Could you check a few things on this model? Use its own coordinates, in mm. Face numbers are marked on the shaded views. A direction names the side the tool comes from. Give positions to 0.01 mm unless a question says otherwise; leave off trailing zeros. Loops run counter-clockwise (first coordinate to the right, second up) from the corner with the lowest first, then second, coordinate; pieces in that order, holes last. Notation, with made-up numbers: (63, -5.75) -> (96, -5.75) arc R17 ccw to (96, -0.75) -> close; hole circle Ø1 at (35, 51.25). An arc over 180 degrees is marked (long way). Write item = value, one per line. Start each with the question number.
1) I'm going to push flat-ended pins straight in: pin 1 Ø3 at (x, z) = (2, -6) entering from +Y; pin 2 Ø2 at (y, z) = (2.5, 2) entering from +X; pin 3 Ø4 at (x, z) = (0.5, 3) entering from +Y. Where does each tip first touch, or does it pass through?
2) I want a section at B-B (x = 0). List the corners of the cut face in (y, z) for me (3 decimals).
3) I want a section at A-A (z = 1). List the corners of the cut face in (x, y) for me (3 decimals), and give its area (3 significant figures).
4) I need wall thicknesses on probe 1 along Y at (x, z) = (0, -0.5) (3 decimals); probe 2 along Z at (x, y) = (-2.5, -2.25); probe 3 along X at (y, z) = (0, 3.5). Which ranges of each line are inside material? Lowest first, please. Write a range as from..to.
5) On a 3-axis mill with a long thin cutter (end or side, diameter ignored), from which of +Z, -Z, +X, -X, +Y, -Y can I reach the whole of each face in a straight line? I mean the marked faces 1, 2 and 3. Say none if no direction works.
6) I want a section at D-D (z = -6). List the corners of the cut face in (x, y) for me (3 decimals), and give its area (3 significant figures).
7) If we mould it in two halves opening along Y, with no side actions, what happens to the marked faces 4, 5 and 6? For each: +Y half, -Y half, draft (parallel to the pull), parting line (faces both ways), or undercut.
8) I want a section at C-C (x = 2.75). List the corners of the cut face in (y, z) for me.
from build123d import *

# Parameters (mm, degrees)
SALIENTE_EXTRUIR1_DEPTH = 3
CROQUIS5_R              = 2.9
SALIENTE_EXTRUIR2_DEPTH = 7.5
CROQUIS4_R              = 0.875
CORTAR_EXTRUIR1_DEPTH   = 10.5


with BuildPart() as part:
    # Croquis1 → Saliente-Extruir1 (new body)
    with BuildSketch(Plane.XY):
        Polygon((-2.057275574, -3.478642055), (1.983954604, -3.520973937), (4.041230177, -0.042331882), (2.057275574, 3.478642055), (-1.983954604, 3.520973937), (-4.041230177, 0.042331882), align=None)
    extrude(amount=SALIENTE_EXTRUIR1_DEPTH)

    # Croquis3 → Revolución1 (revolve)
    with BuildSketch(Plane(origin=(0, 0, 0), x_dir=(1, 0, 0), z_dir=(0, 1, 0))):
        Polygon((-0.5, -5), (-0.75, -5), (-2.5, -3), (-0.5, -3), align=None)
    revolve(axis=Axis((0, 0, 0), (0, 0, 1)))

    # Croquis5 → Saliente-Extruir2 (add)
    with BuildSketch(Plane(origin=(0, 0, 0), x_dir=(-1, 0, 0), z_dir=(0, 0, -1))):
        Circle(CROQUIS5_R)
    extrude(amount=SALIENTE_EXTRUIR2_DEPTH)

    # Croquis4 → Cortar-Extruir1 (cut)
    with BuildSketch(Plane.XY.offset(3)):
        Circle(CROQUIS4_R)
    extrude(amount=-CORTAR_EXTRUIR1_DEPTH, mode=Mode.SUBTRACT)


solid = part.part
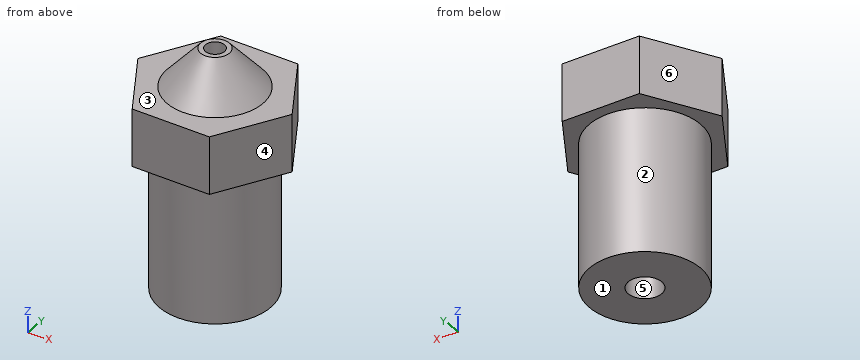
Answer list:
q1.pin_1 = 2.86
q1.pin_2 = 3.17
q1.pin_3 = 3.52
q2.outline = (-3.5, 0) -> (-2.9, 0) -> (-2.9, -7.5) -> (-0.875, -7.5) -> (-0.875, 3) -> (-0.5, 3) -> (-0.5, 5) -> (-0.75, 5) -> (-2.5, 3) -> (-3.5, 3) -> close; (0.5, 3) -> (0.875, 3) -> (0.875, -7.5) -> (2.9, -7.5) -> (2.9, 0) -> (3.5, 0) -> (3.5, 3) -> (2.5, 3) -> (0.75, 5) -> (0.5, 5) -> close
q3.outline = (-4.041, 0.042) -> (-2.057, -3.479) -> (1.984, -3.521) -> (4.041, -0.042) -> (2.057, 3.479) -> (-1.984, 3.521) -> close; hole circle Ø1.75 at (0, 0)
q3.area = 40.0 mm^2
q4.probe_1 = -2.9..-0.875, 0.875..2.9
q4.probe_2 = 0..3
q4.probe_3 = -2.06..-0.5, 0.5..2.06
q5.face_1 = -Z, +X, -X, +Y, -Y
q5.face_2 = -Z
q5.face_3 = +Z
q6.outline = circle Ø5.8 at (0, 0); hole circle Ø1.75 at (0, 0)
q6.area = 24.0 mm^2
q7.face_4 = -Y half
q7.face_5 = undercut
q7.face_6 = +Y half
q8.outline = (-2.23, 0) -> (-0.92, 0) -> (-0.92, -7.5) -> (0.92, -7.5) -> (0.92, 0) -> (2.25, 0) -> (2.25, 3) -> (-2.23, 3) -> close
